Check sheet for the modelled part. Datum: model origin and axes. Units: mm. A direction names the side the tool comes from. Give positions to 0.01 mm unless a question says otherwise; leave off trailing zeros. Write each loop counter-clockwise with the first axis right and the second up, starting at its lowest first coordinate (ties: lowest second). Pieces come first, ordered by that corner, then holes. Notation, with made-up numbers: (48.25, 49) -> (95.25, 49) arc R15 ccw to (95.25, 64) -> close; hole circle Ø11 at (21.5, -27.5). An arc over 180 degrees is marked (long way). Use a Markdown table: item, result. Add a question column.
1. Release check for a two-part mould opening along X. For faces 1 (the flat face through (0, 10, -1)), 2 (the flat face through (0, 8, -1)), 3 (the flat face through (10, 0, -1)) record: released by +X, released by -X, zero draft, split by the parting line, or undercut.
2. Cross-section at A-A (x = -5.5). Enter the section's corners in (y, z).
3. Cross-section at C-C (z = 55). Enter the section's corners in (x, y), then the cut area to 3 significant figures.
4. Gauge pin test, flat end, axial feed: P1, Ø12, axis at x = -6, y = -3.5, coming from the -Z side. Record the tip position at first contact, or that the pin passes through.
5. Scan line: probe 1 along X at (y, z) = (-2, 76.5). Record every from-to range of solid material in increasing order. Write a range as [from, to].
6. Set-up check for faces 4 (the flat face through (-9, 0, 100)), 5 (the flat face through (0, -8, -1)): record each of +Z, -Z, +X, -X, +Y, -Y from which the full face is reachable in a straight line by a thin tool's end or side.
Autodesk Inventor part; units mm, degrees
sketch "Esboço1" plane through (0, 0, 0) normal (0, 0, 1) x (1, 0, 0)
  line L0 (-10, -10) -> (10, -10)
  line L1 (10, -10) -> (10, 10)
  line L2 (10, 10) -> (-10, 10)
  line L3 (-10, 10) -> (-10, -10)
  line L4 (-10, -10) -> (10, 10) construction
  line L5 (10, -10) -> (-10, 10) construction
  line L6 (-8, -8) -> (8, -8)
  line L7 (8, -8) -> (8, 8)
  line L8 (8, 8) -> (-8, 8)
  line L9 (-8, 8) -> (-8, -8)
  line L10 (-8, -8) -> (8, 8) construction
  line L11 (8, -8) -> (-8, 8) construction
  point P0 (0, 0)
  dimension "d0" = 20
  dimension "d1" = 2
extrude "Extrusão1" add sketch "Esboço1" along normal mid plane 200
properties part number "Sessao8_07_04_2025_0002_0001" material "Titânio"
Worked answers:
| question | item | result |
|---|---|---|
| 1 | face 1 | zero draft |
| 1 | face 2 | undercut |
| 1 | face 3 | released by +X |
| 2 | outline | (-10, -100) -> (-8, -100) -> (-8, 100) -> (-10, 100) -> close; (8, -100) -> (10, -100) -> (10, 100) -> (8, 100) -> close |
| 3 | outline | (-10, -10) -> (10, -10) -> (10, 10) -> (-10, 10) -> close; hole (-8, -8) -> (8, -8) -> (8, 8) -> (-8, 8) -> close |
| 3 | area | 144 mm² |
| 4 | P1 | stops at z = -100 |
| 5 | probe 1 | x = [-10, -8], [8, 10] |
| 6 | face 4 | +Z, +X, -X, +Y, -Y |
| 6 | face 5 | +Z, -Z |
